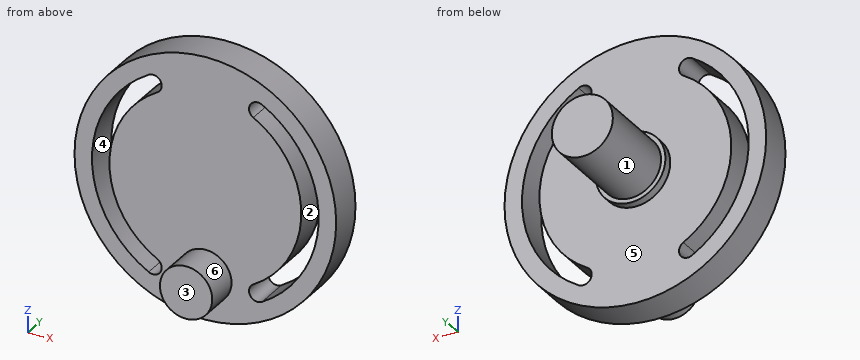
Solid Edge part; units mm, degrees
sketch "Sketch1" plane through (0, 0, 0) normal (0, -1, 0) x (1, 0, 0)
  circle A0 centre (0, 0) radius 75
  arc A1 (-32.5, 56.2917) -> (-27.5, 47.6314) centre (-30, 51.9615) cw
  arc A2 (-27.5, 47.6314) -> (-27.5, -47.6314) centre (0, 0) ccw
  arc A3 (-27.5, -47.6314) -> (-32.5, -56.2917) centre (-30, -51.9615) cw
  arc A4 (-32.5, 56.2917) -> (-32.5, -56.2917) centre (0, 0) ccw
  arc A5 (27.5, 47.6314) -> (32.5, 56.2917) centre (30, 51.9615) cw
  arc A6 (32.5, 56.2917) -> (32.5, -56.2917) centre (0, 0) cw
  arc A7 (32.5, -56.2917) -> (27.5, -47.6314) centre (30, -51.9615) cw
  arc A8 (27.5, 47.6314) -> (27.5, -47.6314) centre (0, 0) cw
extrude "ExtrudedProtrusion_1" add sketch "Sketch1" along normal blind 20
sketch "Sketch2" plane through (0, -20, 0) normal (0, -1, 0) x (1, 0, 0)
  circle A0 centre (0, -50) radius 15
extrude "ExtrudedProtrusion_2" add sketch "Sketch2" along normal blind 20
sketch "Sketch3" plane through (0, 0, 0) normal (0, 1, 0) x (0, 0, -1)
  circle A0 centre (0, 0) radius 20
extrude "ExtrudedProtrusion_3" add sketch "Sketch3" along normal blind 5
sketch "Sketch4" plane through (0, 5, 0) normal (0, 1, 0) x (0, 0, -1)
  circle A0 centre (0, 0) radius 17.5
extrude "ExtrudedProtrusion_4" add sketch "Sketch4" along normal blind 50
Source: CAD feature listing. Evaluate the final solid. Frame: model axes, mm. Face numbers are marked on the shaded views. A direction names the side the tool comes from. Give positions to 0.01 mm unless a question says otherwise; leave off trailing zeros. Write each loop counter-clockwise with the first axis right and the second up, starting at its lowest first coordinate (ties: lowest second). Pieces come first, ordered by that corner, then holes. Notation, with made-up numbers: M -37.75,8.5 L -16.75,8.5 A14 cw -16.75,32.5 Z; hole C 20.5,73 d3. An arc over 180 degrees is marked long. Return JSON: item names as keys, results as strings. Group by question number.
1) Pull-direction query (Z, two-part tool) for the marked faces 4, 5 and 6; classes: pulls with the +Z half, pulls with the -Z half, needs draft (parallel to the pull), parting line crosses it, or undercut.
2) Cut plane A-A, the plane z = 0. Output: boundary loops of the cut face in (x, y).
3) Pin query (flat end, axial travel): P1, Ø1.5, axis at x = -38, y = -9.5, coming from the -Z side; P2, Ø12, axis at x = 18.5, y = 23.5, coming from the -Z side; P3, Ø10, axis at x = -18, y = -12.5, coming from the -Z side. Return the tip coordinate at first contact, or that it passes through.
4) Material intervals for line 1 along X through (y, z) = (-10, 42); line 2 along X through (y, z) = (-19.5, -14); line 3 along Z through (x, y) = (-39, -14), sorted ascending. Write a range as [from, to].
5) Set-up query: the marked faces 1, 2 and 3. Return all of +Z, -Z, +X, -X, +Y, -Y with unobstructed straight access to the full face (end or side cutting, diameter ignored); none if empty.
6) Cut plane B-B, the plane x = 43. Output: boundary loops of the cut face in (y, z).
7) Cut plane D-D, the plane z = -39.5. Output: boundary loops of the cut face in (x, y).
8) Cut plane C-C, the plane y = -16.5. Output: boundary loops of the cut face in (x, z).
Recorded:
{
 "1": {"face 4": "undercut", "face 5": "needs draft", "face 6": "parting line crosses it"},
 "2": {"outline": "M -75,-20 L -65,-20 L -65,0 L -75,0 Z; M -55,-20 L 55,-20 L 55,0 L 20,0 L 20,5 L 17.5,5 L 17.5,55 L -17.5,55 L -17.5,5 L -20,5 L -20,0 L -55,0 Z; M 65,-20 L 75,-20 L 75,0 L 65,0 Z"},
 "3": {"P1": "stops at z = -65.1", "P2": "stops at z = -12.25", "P3": "stops at z = -73.86"},
 "4": {"line 1": "x = [-62.14, -49.61], [-35.51, 35.51], [49.61, 62.14]", "line 2": "x = [-73.68, -63.47], [-53.19, 53.19], [63.47, 73.68]", "line 3": "z = [-64.06, -52], [-38.78, 38.78], [52, 64.06]"},
 "5": {"face 1": "+Y", "face 2": "+Y, -Y", "face 3": "+Z, -Z, +X, -X, -Y"},
 "6": {"outline": "M -20,-61.45 L 0,-61.45 L 0,-48.74 L -20,-48.74 Z; M -20,-34.29 L 0,-34.29 L 0,34.29 L -20,34.29 Z; M -20,48.74 L 0,48.74 L 0,61.45 L -20,61.45 Z"},
 "7": {"outline": "M -63.76,-20 L -51.62,-20 L -51.62,0 L -63.76,0 Z; M -38.27,-20 L -10.71,-20 L -10.71,-40 L 10.71,-40 L 10.71,-20 L 38.27,-20 L 38.27,0 L -38.27,0 Z; M 51.62,-20 L 63.76,-20 L 63.76,0 L 51.62,0 Z"},
 "8": {"outline": "C 0,0 d150; hole M -32.5,-56.29 A5 ccw -27.5,-47.63 A55 cw -27.5,47.63 A5 ccw -32.5,56.29 A65 ccw Z; hole M 27.5,-47.63 A5 ccw 32.5,-56.29 A65 ccw 32.5,56.29 A5 ccw 27.5,47.63 A55 cw Z"}
}
